from build123d import *

# Parameters (mm, degrees)
SKETCH_1_W          = 35
SKETCH_1_H          = 35
SKETCH_1_R          = 4.5
SKETCH_1_R_2        = 2.15
EXTRUDE_1_DEPTH     = 25
FILLET_1_R          = 5
SKETCH_3_R          = 6.1
CUT_EXTRUDE_1_DEPTH = 4
SKETCH_4_R          = 6.1
CUT_EXTRUDE_2_DEPTH = 4
SKETCH_6_R          = 10
CUT_EXTRUDE_3_DEPTH = 9
SKETCH_7_W          = 9
SKETCH_7_H          = 9
CUT_EXTRUDE_4_DEPTH = 15
FILLET_3_R          = 2
CHAMFER_1_SIZE      = 1
CHAMFER_2_SIZE      = 0.5


with BuildPart() as part:
    # 草图1 → 凸台-拉伸1 (new body)
    with BuildSketch(Plane(origin=(0, 0, 0), x_dir=(1, 0, 0), z_dir=(0, 1, 0))):
        Rectangle(SKETCH_1_W, SKETCH_1_H)
        with Locations(Location((0, 0, 0), (0, 0, 270))):
            Circle(SKETCH_1_R, mode=Mode.SUBTRACT)
        with Locations(Location((13, 13, 0), (0, 0, 270))):
            Circle(SKETCH_1_R_2, mode=Mode.SUBTRACT)
        with Locations(Location((13, -13, 0), (0, 0, 270))):
            Circle(SKETCH_1_R_2, mode=Mode.SUBTRACT)
        with Locations(Location((-13, -13, 0), (0, 0, 270))):
            Circle(SKETCH_1_R_2, mode=Mode.SUBTRACT)
        with Locations(Location((-13, 13, 0), (0, 0, 270))):
            Circle(SKETCH_1_R_2, mode=Mode.SUBTRACT)
    extrude(amount=EXTRUDE_1_DEPTH)

    # 圆角1
    fillet_1_edges = [part.edges().sort_by_distance(p)[0] for p in [
        (17.5, 12.5, 17.5),
        (-17.5, 12.5, 17.5),
        (-17.5, 12.5, -17.5),
        (17.5, 12.5, -17.5),
    ]]
    fillet(fillet_1_edges, radius=FILLET_1_R)

    # 草图3 → 切除-拉伸1 (cut)
    with BuildSketch(Plane(origin=(0, 25, 0), x_dir=(1, 0, 0), z_dir=(0, 1, 0))):
        with Locations(Location((0, 0, 0), (0, 0, 270))):
            Circle(SKETCH_3_R)
    extrude(amount=-CUT_EXTRUDE_1_DEPTH, mode=Mode.SUBTRACT)

    # 草图4 → 切除-拉伸2 (cut)
    with BuildSketch(Plane(origin=(0, 13, 0), x_dir=(1, 0, 0), z_dir=(0, 1, 0))):
        with Locations(Location((0, 0, 0), (0, 0, 270))):
            Circle(SKETCH_4_R)
    extrude(amount=-CUT_EXTRUDE_2_DEPTH, mode=Mode.SUBTRACT)

    # 草图6 → 切除-拉伸3 (cut)
    with BuildSketch(Plane.XZ):
        with Locations(Location((0, 0, 0), (0, 0, 270))):
            Circle(SKETCH_6_R)
    extrude(amount=-CUT_EXTRUDE_3_DEPTH, mode=Mode.SUBTRACT)

    # 草图7 → 切除-拉伸4 (cut)
    with BuildSketch(Plane(origin=(0, 25, 0), x_dir=(1, 0, 0), z_dir=(0, 1, 0))):
        with Locations((-13, 13)):
            Rectangle(SKETCH_7_W, SKETCH_7_H)
        with Locations((13, 13)):
            Rectangle(SKETCH_7_W, SKETCH_7_H)
        with Locations((13, -13)):
            Rectangle(SKETCH_7_W, SKETCH_7_H)
        with Locations((-13, -13)):
            Rectangle(SKETCH_7_W, SKETCH_7_H)
    extrude(amount=-CUT_EXTRUDE_4_DEPTH, mode=Mode.SUBTRACT)

    # 圆角3
    fillet_3_edges = [part.edges().sort_by_distance(p)[0] for p in [
        (-17.5, 17.5, 8.5),
        (-8.5, 17.5, 8.5),
        (-8.5, 17.5, 17.5),
        (8.5, 17.5, 17.5),
        (8.5, 17.5, 8.5),
        (17.5, 17.5, 8.5),
        (17.5, 17.5, -8.5),
        (8.5, 17.5, -8.5),
        (8.5, 17.5, -17.5),
        (-8.5, 17.5, -17.5),
        (-8.5, 17.5, -8.5),
        (-17.5, 17.5, -8.5),
    ]]
    fillet(fillet_3_edges, radius=FILLET_3_R)

    # 倒角1
    chamfer_1_edges = [part.edges().sort_by_distance(p)[0] for p in [
        (0, 0, 10),
    ]]
    chamfer(chamfer_1_edges, length=CHAMFER_1_SIZE)

    # 倒角2
    chamfer_2_edges = [part.edges().sort_by_distance(p)[0] for p in [
        (0, 21, -4.5),
        (0, 13, -4.5),
    ]]
    chamfer(chamfer_2_edges, length=CHAMFER_2_SIZE)


solid = part.part
Input: part model. Units: mm. Frame: model coordinates. A direction names the side the tool comes from. Coordinates: 2 decimals unless noted, no trailing zeros. Loops run counter-clockwise (first coordinate to the right, second up) from the corner with the lowest first, then second, coordinate; pieces in that order, holes last. Notation, with made-up numbers: (-28.5, 28.5) -> (18.5, 28.5) arc R29 cw to (18.5, 61.5) -> close; hole circle Ø5 at (20, -26.5). An arc over 180 degrees is marked (long way). Write each question's results on one line, items separated by ' | '. Start each with the question number.
Q1. Section B-B, the plane x = 0. Return the cut outline in (y, z).
Q2. Pull-direction query (X, two-part tool) for faces 4 (the flat face through (13.1, 10, 10.7)), 5 (the cylindrical face through (11.09, 4.93, 13.99)), 6 (the flat face through (-8.5, 18, -13)), 7 (the cylindrical face through (9.1, 17.4, 9.07)); classes: released by +X, released by -X, zero draft, split by the parting line, or undercut.
Q3. Section A-A, the plane z = 0. Return the cut outline in (x, y), plus the area to 3 significant figures.
Q4. Reachability of faces 1 (the flat face through (-15, 10, -15)), 2 (the cylindrical face through (-3.71, 11.03, -4.84)), 3 (the cylindrical face through (-7.9, 17.4, 16.93)) from +Z, -Z, +X, -X, +Y, -Y: full face, straight path, thin tool, end or side. Return the list, or none.
Q5. Ray query, line 1 (X direction, y = 11.75, z = 0); line 2 (X direction, y = 18.75, z = 0); line 3 (X direction, y = 4.25, z = -13). Return the intervals inside material, ascending. Write a range as from..to.
Q6. Pin query (flat end, axial travel): pin 1 (3 mm diameter, centred on x = 9.5, y = 19.5, fed in from +Z); pin 2 (6 mm diameter, centred on x = 5, z = -11.5, fed in from -Y); pin 3 (2.5 mm diameter, centred on x = -12, y = 14.5, fed in from -Z); pin 4 (5.5 mm diameter, centred on y = 16.5, z = 12.5, fed in from -X). Return the tip coordinate at first contact, or that it passes through.
Q7. Section D-D, the plane y = 2.75. Return the cut outline in (x, z), plus the area to 3 significant figures.
Q8. Section C-C, the plane y = 12. Return the cut outline in (x, z), plus the area to 3 significant figures.
Found:
1) outline: (0, -17.5) -> (25, -17.5) -> (25, -6.1) -> (21, -6.1) -> (21, -5) -> (20.5, -4.5) -> (13.5, -4.5) -> (13, -5) -> (13, -6.1) -> (9, -6.1) -> (9, -10) -> (1, -10) -> (0, -11) -> close; (0, 11) -> (1, 10) -> (9, 10) -> (9, 6.1) -> (13, 6.1) -> (13, 5) -> (13.5, 4.5) -> (20.5, 4.5) -> (21, 5) -> (21, 6.1) -> (25, 6.1) -> (25, 17.5) -> (0, 17.5) -> close
2) face 4: zero draft | face 5: undercut | face 6: released by -X | face 7: released by +X
3) outline: (-17.5, 0) -> (-11, 0) -> (-10, 1) -> (-10, 9) -> (-6.1, 9) -> (-6.1, 13) -> (-5, 13) -> (-4.5, 13.5) -> (-4.5, 20.5) -> (-5, 21) -> (-6.1, 21) -> (-6.1, 25) -> (-17.5, 25) -> close; (4.5, 13.5) -> (5, 13) -> (6.1, 13) -> (6.1, 9) -> (10, 9) -> (10, 1) -> (11, 0) -> (17.5, 0) -> (17.5, 25) -> (6.1, 25) -> (6.1, 21) -> (5, 21) -> (4.5, 20.5) -> close | area: 524 mm2
4) face 1: -Z, -X, +Y | face 2: -Y | face 3: +Z, -X, +Y
5) line 1: -17.5..-6.1, 6.1..17.5 | line 2: -17.5..-4.5, 4.5..17.5 | line 3: -17.47..-15.15, -10.85..10.85, 15.15..17.47
6) pin 1: z = 16.82 | pin 2: y = 0 | pin 3: z = -8.5 | pin 4: x = -8.65
7) outline: (-17.5, -12.5) arc R5 ccw to (-12.5, -17.5) -> (12.5, -17.5) arc R5 ccw to (17.5, -12.5) -> (17.5, 12.5) arc R5 ccw to (12.5, 17.5) -> (-12.5, 17.5) arc R5 ccw to (-17.5, 12.5) -> close; hole circle Ø4.3 at (-13, -13); hole circle Ø4.3 at (-13, 13); hole circle Ø20 at (0, 0); hole circle Ø4.3 at (13, -13); hole circle Ø4.3 at (13, 13) | area: 831 mm2
8) outline: (-17.5, -6.5) arc R2 ccw to (-15.5, -8.5) -> (-10.5, -8.5) arc R2 cw to (-8.5, -10.5) -> (-8.5, -15.5) arc R2 ccw to (-6.5, -17.5) -> (6.5, -17.5) arc R2 ccw to (8.5, -15.5) -> (8.5, -10.5) arc R2 cw to (10.5, -8.5) -> (15.5, -8.5) arc R2 ccw to (17.5, -6.5) -> (17.5, 6.5) arc R2 ccw to (15.5, 8.5) -> (10.5, 8.5) arc R2 cw to (8.5, 10.5) -> (8.5, 15.5) arc R2 ccw to (6.5, 17.5) -> (-6.5, 17.5) arc R2 ccw to (-8.5, 15.5) -> (-8.5, 10.5) arc R2 cw to (-10.5, 8.5) -> (-15.5, 8.5) arc R2 ccw to (-17.5, 6.5) -> close; hole circle Ø12.2 at (0, 0) | area: 781 mm2
